For this review, take the finished solid that the model builds, in its own axes (mm). A direction names the side the tool comes from. Round coordinates to 2 decimals unless told otherwise and drop trailing zeros. Write each loop counter-clockwise with the first axis right and the second up, starting at its lowest first coordinate (ties: lowest second). Pieces come first, ordered by that corner, then holes. Notation, with made-up numbers: M 27.25,59 L 40.25,59 A5 cw 40.25,63 Z; hole C -37.5,-13 d10. An arc over 180 degrees is marked long. Write each question's results on one line, items separated by ' | '. Start each with the question number.
```python
from build123d import *

# Parameters (mm, degrees)
BOSS_EXTRUDE1_DEPTH = 4.35
FILLET1_R           = 0.25


with BuildPart() as part:
    # Sketch1 → Boss-Extrude1 (new body, symmetric)
    with BuildSketch(Plane.XY):
        Polygon((-4.5, 2.7), (-4.5, -2.7), (4.5, -2.7), (4.5, 2.7), (3.45, 2.7), (3.45, -1), (2.5125, -1), (2.5125, 2.7), (1.4625, 2.7), (1.4625, -1), (0.525, -1), (0.525, 2.7), (-0.525, 2.7), (-0.525, -1), (-1.4625, -1), (-1.4625, 2.7), (-2.5125, 2.7), (-2.5125, -1), (-3.45, -1), (-3.45, 2.7), align=None)
    extrude(amount=BOSS_EXTRUDE1_DEPTH, both=True)

    # Fillet1
    fillet1_edges = [part.edges().sort_by_distance(p)[0] for p in [
        (-3.45, 2.7, 0),
        (-3.45, -1, 0),
        (-2.5125, -1, 0),
        (-2.5125, 2.7, 0),
        (-1.4625, 2.7, 0),
        (-1.4625, -1, 0),
        (-0.525, -1, 0),
        (-0.525, 2.7, 0),
        (0.525, 2.7, 0),
        (0.525, -1, 0),
        (1.4625, -1, 0),
        (1.4625, 2.7, 0),
        (2.5125, 2.7, 0),
        (2.5125, -1, 0),
        (3.45, -1, 0),
        (3.45, 2.7, 0),
        (4.5, 2.7, 0),
        (4.5, -2.7, 0),
        (-4.5, -2.7, 0),
        (-4.5, 2.7, 0),
    ]]
    fillet(fillet1_edges, radius=FILLET1_R)


solid = part.part
```
Item 1: Insertion check: P1, Ø0.5, axis at x = 1, z = -1, coming from the +Y side. The pin has a flat end and moves straight along its axis. Give the tip position at first contact, or say it passes through.
Item 2: For probe 1 along Y at (x, z) = (2.75, 1), list the stretches that pass through material, from the lowest coordinate up.
Item 3: Mouldability with a two-part tool opening along X and no side actions: class faces 3 (the flat face through (4.5, 0, 0)), 4 (the flat face through (-2.512, 1, 0)), 5 (the flat face through (-0.525, 1, 0)), 6 (the flat face through (0, -1, -4.35)) as pulls with the +X half, pulls with the -X half, needs draft (parallel to the pull), parting line crosses it, or undercut.
Item 4: We need section B-B on x = 3. State the section outline as (y, z) points, then the cut area to 3 significant figures.
Item 5: For faces 1 (the flat face through (0.525, 1, 0)), 2 (the flat face through (0, -1, 4.35)), list the 3-axis set-ups (+Z, -Z, +X, -X, +Y, -Y) from which the entire face can be reached by the end or side of a thin tool; tool diameter is ignored.
Item 6: We need section A-A on y = 0.4. State how many separate pieces and enclosed holes the cut face has, then the cut area to 3 significant figures.
Numbers:
1) P1: stops at y = -1
2) probe 1: y = -2.7 to -1
3) face 3: pulls with the +X half | face 4: undercut | face 5: undercut | face 6: needs draft
4) outline: M -2.7,-4.35 L -1,-4.35 L -1,4.35 L -2.7,4.35 Z | area: 14.8 mm^2
5) face 1: +Z, -Z, +Y | face 2: +Z, +X, -X, +Y, -Y
6) separate pieces: 5 | enclosed holes: 0 | area: 45.7 mm^2
